```python
from build123d import *

# Parameters (mm, degrees)
SKETCH1_R                      = 2
BOSS_EXTRUDE1_DEPTH            = 6
CUT_EXTRUDE1_DEPTH             = 3.9
BOSS_EXTRUDE2_DEPTH            = 138.475201729
BOSS_EXTRUDE3_DEPTH            = 8
CUT_EXTRUDE2_REACH             = 160.595
SKETCH5_R                      = 2
CUT_EXTRUDE2_DIRECTION_2_DEPTH = 159.594869272
CUT_EXTRUDE3_DEPTH             = 3.9


with BuildPart() as part:
    # Sketch1 → Boss-Extrude1 (new body)
    with BuildSketch(Plane.XY):
        Polygon((0, 17), (0, -17), (-10, -27), (-28.499995142, -45.499995142), (-46.999990284, -27), (-46.646446609, 27), (-28.323223305, 45.323223305), (-10, 27), align=None)
        with Locations((-10, -8)):
            Circle(SKETCH1_R, mode=Mode.SUBTRACT)
        with Locations((-10, 8)):
            Circle(SKETCH1_R, mode=Mode.SUBTRACT)
    extrude(amount=BOSS_EXTRUDE1_DEPTH)

    # Sketch2 → Cut-Extrude1 (cut)
    with BuildSketch(Plane.XY.offset(6)):
        Polygon((-10, 11.983716857), (-13.45, 9.991858429), (-13.45, 6.008141571), (-10, 4.016283143), (-6.55, 6.008141571), (-6.55, 9.991858429), align=None)
        Polygon((-10, -4.016283143), (-13.45, -6.008141571), (-13.45, -9.991858429), (-10, -11.983716857), (-6.55, -9.991858429), (-6.55, -6.008141571), align=None)
    extrude(amount=-CUT_EXTRUDE1_DEPTH, mode=Mode.SUBTRACT)

    # Sketch3 → Boss-Extrude2 (add)
    with BuildSketch(Plane.XY.offset(6)):
        Polygon((-28.499995142, -39.136034112), (-4.5, -15.136038969), (-4.5, 15.136038969), (-28.323223305, 38.959262274), (-31.50520382, 42.141242789), (-28.323223305, 45.323223305), (0, 17), (0, -17), (-28.499995142, -45.499995142), (-31.681975658, -42.318014627), align=None)
    extrude(amount=BOSS_EXTRUDE2_DEPTH)

    # Sketch4 → Boss-Extrude3 (add)
    with BuildSketch(Plane.XY.offset(144.475201729)):
        Polygon((0, 17), (0, -17), (-28.499995142, -45.499995142), (-46.999990284, -27), (-46.646446609, 27), (-28.323223305, 45.323223305), align=None)
    extrude(amount=-BOSS_EXTRUDE3_DEPTH)

    # Sketch5 → Cut-Extrude2 (cut, up to next)
    with BuildSketch(Plane.XY.offset(144.475201729), mode=Mode.PRIVATE) as cut_extrude2_sk1:
        with Locations(Location((-27.938888553, -23.433684733, 0), (0, 0, 180))):
            Circle(SKETCH5_R)
    cut_extrude2_tool1 = extrude(cut_extrude2_sk1.sketch, amount=-CUT_EXTRUDE2_REACH, mode=Mode.PRIVATE) & part.part
    # Sketch5 → Cut-Extrude2 (cut, up to next)
    with BuildSketch(Plane.XY.offset(144.475201729), mode=Mode.PRIVATE) as cut_extrude2_sk2:
        with Locations(Location((-27.762116716, 23.256912896, 0), (0, 0, 180))):
            Circle(SKETCH5_R)
    cut_extrude2_tool2 = extrude(cut_extrude2_sk2.sketch, amount=-CUT_EXTRUDE2_REACH, mode=Mode.PRIVATE) & part.part
    # Sketch5 → Cut-Extrude2 (cut, up to next)
    with BuildSketch(Plane.XY.offset(144.475201729), mode=Mode.PRIVATE) as cut_extrude2_sk3:
        with Locations(Location((-38.875423831, -8, 0), (0, 0, 180))):
            Circle(SKETCH5_R)
    cut_extrude2_tool3 = extrude(cut_extrude2_sk3.sketch, amount=-CUT_EXTRUDE2_REACH, mode=Mode.PRIVATE) & part.part
    # Sketch5 → Cut-Extrude2 (cut, up to next)
    with BuildSketch(Plane.XY.offset(144.475201729), mode=Mode.PRIVATE) as cut_extrude2_sk4:
        with Locations(Location((-38.875423831, 8, 0), (0, 0, 180))):
            Circle(SKETCH5_R)
    cut_extrude2_tool4 = extrude(cut_extrude2_sk4.sketch, amount=-CUT_EXTRUDE2_REACH, mode=Mode.PRIVATE) & part.part
    add(cut_extrude2_tool1.solids().sort_by_distance((-27.938889, -23.433685, 144.475202))[0], mode=Mode.SUBTRACT)
    add(cut_extrude2_tool2.solids().sort_by_distance((-27.762117, 23.256913, 144.475202))[0], mode=Mode.SUBTRACT)
    add(cut_extrude2_tool3.solids().sort_by_distance((-38.875424, -8, 144.475202))[0], mode=Mode.SUBTRACT)
    add(cut_extrude2_tool4.solids().sort_by_distance((-38.875424, 8, 144.475202))[0], mode=Mode.SUBTRACT)

    # Sketch5 → Cut-Extrude2 direction 2 (cut)
    with BuildSketch(Plane.XY.offset(144.475201729)):
        with Locations(Location((-27.938888553, -23.433684733, 0), (0, 0, 180))):
            Circle(SKETCH5_R)
        with Locations(Location((-27.762116716, 23.256912896, 0), (0, 0, 180))):
            Circle(SKETCH5_R)
        with Locations(Location((-38.875423831, -8, 0), (0, 0, 180))):
            Circle(SKETCH5_R)
        with Locations(Location((-38.875423831, 8, 0), (0, 0, 180))):
            Circle(SKETCH5_R)
    extrude(amount=CUT_EXTRUDE2_DIRECTION_2_DEPTH, mode=Mode.SUBTRACT)

    # Sketch6 → Cut-Extrude3 (cut)
    with BuildSketch(Plane.XY.offset(144.475201729)):
        Polygon((-27.762116716, 27.240629753), (-31.212116716, 25.248771324), (-31.212116716, 21.265054467), (-27.762116716, 19.273196038), (-24.312116716, 21.265054467), (-24.312116716, 25.248771324), align=None)
        Polygon((-38.875423831, 11.983716857), (-42.325423831, 9.991858429), (-42.325423831, 6.008141571), (-38.875423831, 4.016283143), (-35.425423831, 6.008141571), (-35.425423831, 9.991858429), align=None)
        Polygon((-38.875423831, -4.016283143), (-42.325423831, -6.008141571), (-42.325423831, -9.991858429), (-38.875423831, -11.983716857), (-35.425423831, -9.991858429), (-35.425423831, -6.008141571), align=None)
        Polygon((-27.938888553, -19.449967876), (-31.388888553, -21.441826304), (-31.388888553, -25.425543162), (-27.938888553, -27.417401591), (-24.488888553, -25.425543162), (-24.488888553, -21.441826304), align=None)
    extrude(amount=-CUT_EXTRUDE3_DEPTH, mode=Mode.SUBTRACT)


solid = part.part
```
For this review, take the finished solid that the model builds, in its own axes (mm). A direction names the side the tool comes from. Give positions to 0.01 mm unless a question says otherwise; leave off trailing zeros. Write each loop counter-clockwise with the first axis right and the second up, starting at its lowest first coordinate (ties: lowest second). Pieces come first, ordered by that corner, then holes.
Item 1: Take a section at B-B (y = 8). Give the boundary of the cut face in (x, z), and give its area (3 significant figures).
Item 2: Take a section at D-D (y = -8). Give the boundary of the cut face in (x, z).
Item 3: Take a section at C-C (x = -16). Give the boundary of the cut face in (y, z), and give its area (3 significant figures).
Item 4: The part is to be moulded in two halves that separate along Y. For faces 1 (the face through (-9, 6, 2.1)), 2 (the face through (0, 0, 71)), say which applies: +Y half, -Y half, draft (parallel to the pull), parting line (faces both ways), or undercut.
Item 5: Machinability: for faces 3 (the face through (-37.17, 5, 142.55)), 4 (the face through (-30, 1, 6)), 5 (the face through (-8.3, -5, 4.1)), which of the approach directions +Z, -Z, +X, -X, +Y, -Y give a long, thin tool a straight path to every point of the face, cutting with its end or side? Answer none if there is none.
Item 6: Take a section at A-A (z = 29.5). Give the boundary of the cut face in (x, y).
Item 7: Insertion check: P1, Ø12, axis at x = -35.5, z = 94, coming from the +Y side; P2, Ø6, axis at x = -39.5, y = -14.5, coming from the -Z side; P3, Ø5, axis at x = -29, z = 36.5, coming from the -Y side; P4, Ø2, axis at y = -7, z = 142, coming from the -X side. Each pin has a flat end and moves straight along its axis. Give the tip position at first contact, or say it passes through.
Item 8: Wall thickness on probe 1 along Z at (x, y) = (-39, 0.5); probe 2 along Y at (x, z) = (-10, 1.1); probe 3 along Z at (x, y) = (-37.5, -5): over which ranges is each line inside the solid? List them lowest first.
Established:
1. outline: (-46.77, 0) - (-12, 0) - (-12, 2.1) - (-13.45, 2.1) - (-13.45, 6) - (-46.77, 6) - close; (-46.77, 136.48) - (-40.88, 136.48) - (-40.88, 140.58) - (-42.33, 140.58) - (-42.33, 144.48) - (-46.77, 144.48) - close; (-36.88, 136.48) - (-4.5, 136.48) - (-4.5, 6) - (-6.55, 6) - (-6.55, 2.1) - (-8, 2.1) - (-8, 0) - (0, 0) - (0, 144.48) - (-35.43, 144.48) - (-35.43, 140.58) - (-36.88, 140.58) - close
1. area: 1,160 mm2
2. outline: (-46.88, 0) - (-12, 0) - (-12, 2.1) - (-13.45, 2.1) - (-13.45, 6) - (-46.88, 6) - close; (-46.88, 136.48) - (-40.88, 136.48) - (-40.88, 140.58) - (-42.33, 140.58) - (-42.33, 144.48) - (-46.88, 144.48) - close; (-36.88, 136.48) - (-4.5, 136.48) - (-4.5, 6) - (-6.55, 6) - (-6.55, 2.1) - (-8, 2.1) - (-8, 0) - (0, 0) - (0, 144.48) - (-35.43, 144.48) - (-35.43, 140.58) - (-36.88, 140.58) - close
3. outline: (-33, 0) - (33, 0) - (33, 144.48) - (-33, 144.48) - close; hole (-26.64, 6) - (26.64, 6) - (26.64, 136.48) - (-26.64, 136.48) - close
3. area: 2,580 mm2
4. face 1: undercut
4. face 2: draft
5. face 3: +Z
5. face 4: -X
5. face 5: none
6. outline: (-31.68, -42.32) - (-28.5, -45.5) - (0, -17) - (0, 17) - (-28.32, 45.32) - (-31.51, 42.14) - (-4.5, 15.14) - (-4.5, -15.14) - close
7. P1: stops at y = 44.15
7. P2: stops at z = 0
7. P3: stops at y = -45.5
7. P4: stops at x = -46.88
8. probe 1: z = 0 to 6, 136.48 to 144.48
8. probe 2: y = -27 to -10, -6 to 6, 10 to 27
8. probe 3: z = 0 to 6, 136.48 to 140.58
